Source: CAD feature listing. Evaluate the final solid. Frame: model axes, mm. Coordinates: 2 decimals unless noted, no trailing zeros. One line per question, with ' | ' between items. Start each with the question number.
(1) Contact query for a flat-ended pin moving along its axis: P1, Ø3.5, axis at y = 25.4, z = -220.72, coming from the -X side. Output: stop coordinate, or through.
(2) Line query: line 1 along Y through (x, z) = (1.55, -147.5); line 2 along Y through (x, z) = (0.75, -185); line 3 along Z through (x, y) = (1.75, 48). Output: solid intervals per line, ascending.
(3) Draft query along X for faces 1 (the flat face through (0, 26, -182)), 2 (the flat face through (3.175, 26, -182)). Return one class per face: +X half, -X half, draft (parallel to the pull), parting line (faces both ways), or undercut.
from build123d import *

# Parameters (mm, degrees)
SKETCH1_W           = 368.3
SKETCH1_H           = 50.8
BOSS_EXTRUDE1_DEPTH = 3.175
SKETCH2_R           = 2.032
CUT_EXTRUDE1_DEPTH  = 372.80049842
CHAMFER1_SIZE       = 6.35
FILLET1_R           = 3.175


with BuildPart() as part:
    # Sketch1 → Boss-Extrude1 (new body)
    with BuildSketch(Plane(origin=(0, 0, 0), x_dir=(0, 0, -1), z_dir=(1, 0, 0))):
        with Locations((184.15, 25.4)):
            Rectangle(SKETCH1_W, SKETCH1_H)
    extrude(amount=BOSS_EXTRUDE1_DEPTH)

    # Sketch2 → Cut-Extrude1 (cut, through all)
    with BuildSketch(Plane(origin=(3.175, 0, 0), x_dir=(0, 0, -1), z_dir=(1, 0, 0))):
        with Locations((327.905386247, 25.4)):
            Circle(SKETCH2_R)
        with Locations((291.329386247, 25.4)):
            Circle(SKETCH2_R)
        with Locations((256.023386247, 25.4)):
            Circle(SKETCH2_R)
        with Locations((220.717386247, 25.4)):
            Circle(SKETCH2_R)
        with Locations((184.15, 24.60625)):
            Circle(SKETCH2_R)
        with Locations((147.582613753, 25.4)):
            Circle(SKETCH2_R)
        with Locations((112.276613753, 25.4)):
            Circle(SKETCH2_R)
        with Locations((76.970613753, 25.4)):
            Circle(SKETCH2_R)
        with Locations((40.394613753, 25.4)):
            Circle(SKETCH2_R)
    extrude(amount=-CUT_EXTRUDE1_DEPTH, mode=Mode.SUBTRACT)

    # Chamfer1
    chamfer1_edges = [part.edges().sort_by_distance(p)[0] for p in [
        (1.5875, 0, -368.3),
        (1.5875, 0, 0),
    ]]
    chamfer(chamfer1_edges, length=CHAMFER1_SIZE)

    # Fillet1
    fillet1_edges = [part.edges().sort_by_distance(p)[0] for p in [
        (1.5875, 0, -361.95),
        (1.5875, 0, -6.35),
        (1.5875, 6.35, 0),
        (1.5875, 6.35, -368.3),
        (1.5875, 50.8, 0),
        (1.5875, 50.8, -368.3),
    ]]
    fillet(fillet1_edges, radius=FILLET1_R)


solid = part.part
Response values:
1) P1: passes through
2) line 1: y = 0 to 23.37, 27.43 to 50.8 | line 2: y = 0 to 22.76, 26.45 to 50.8 | line 3: z = -368.28 to -0.02
3) face 1: -X half | face 2: +X half
